Autodesk Inventor part; units mm, degrees
ref_plane "YZ Plane" through (0, 0, 0) normal (1, 0, 0) x (0, 1, 0)
ref_plane "XZ Plane" through (0, 0, 0) normal (0, 1, 0) x (-1, 0, 0)
ref_plane "XY Plane" through (0, 0, 0) normal (0, 0, 1) x (1, 0, 0)
sketch "Skizze1" plane through (0, 0, 0) normal (0, 1, 0) x (-1, 0, 0)
  line L0 (159.3398, 191.458) -> (9.3398, 191.458)
  line L1 (9.3398, 191.458) -> (9.3398, -108.542)
  line L2 (9.3398, -108.542) -> (159.3398, -108.542)
  line L3 (159.3398, -108.542) -> (159.3398, 191.458)
  point P0 (0, 0)
  dimension "d0" = 300
  dimension "d1" = 150
extrude "Extrusion1" add sketch "Skizze1" along normal blind 190
sketch "Skizze2" plane through (0, 190, 0) normal (0, 1, 0) x (1, 0, 0)
  line L0 (-9.3398, 108.542) -> (-159.3398, 108.542)
  line L1 (-159.3398, -191.458) -> (-9.3398, -191.458)
  line L2 (-9.3398, -191.458) -> (-9.3398, 108.542)
  line L3 (-9.3398, 108.542) -> (-159.3398, 108.542)
  line L4 (-159.3398, 108.542) -> (-159.3398, -191.458)
  line L5 (-9.3398, 108.542) -> (-89.3398, 108.542)
  line L6 (-89.3398, 108.542) -> (-89.3398, 48.542)
  line L7 (-69.3398, 28.542) -> (-9.3398, 28.542)
  line L8 (-9.3398, 28.542) -> (-9.3398, 108.542)
  line L9 (-9.3398, -191.458) -> (-9.3398, 108.542)
  line L10 (-9.3398, -191.458) -> (-89.3398, -191.458)
  line L11 (-89.3398, -191.458) -> (-89.3398, -131.458)
  line L12 (-69.3398, -111.458) -> (-9.3398, -111.458)
  line L13 (-9.3398, -111.458) -> (-9.3398, -191.458)
  arc A0 (-69.3398, -111.458) -> (-89.3398, -131.458) centre (-69.3398, -131.458) ccw
  arc A1 (-89.3398, 48.542) -> (-69.3398, 28.542) centre (-69.3398, 48.542) ccw
  point P0 (0, 0)
  point P1 (-89.3398, 28.542)
  point P2 (-89.3398, -111.458)
  dimension "d4" = 80
  dimension "d5" = 80
  dimension "d6" = 80
  dimension "d7" = 80
  dimension "d8" = 20
  dimension "d9" = 20
extrude "Extrusion2" cut sketch "Skizze2" against normal blind 20 contours L2 L7 A1 L6 L0 | L2 L1 L11 A0 L12
sketch "Skizze3" plane through (0, 170, 0) normal (0, 1, 0) x (1, 0, 0)
  line L0 (-9.3398, -111.458) -> (-9.3398, -191.458)
  line L1 (-69.3398, -111.458) -> (-9.3398, -111.458)
  arc A0 (-69.3398, -111.458) -> (-89.3398, -131.458) centre (-69.3398, -131.458) ccw
  line L2 (-89.3398, -191.458) -> (-89.3398, -131.458)
  line L3 (-9.3398, -191.458) -> (-89.3398, -191.458)
  line L4 (-9.3398, 108.542) -> (-9.3398, 28.542)
  line L5 (-89.3398, 108.542) -> (-9.3398, 108.542)
  line L6 (-89.3398, 48.542) -> (-89.3398, 108.542)
  arc A1 (-89.3398, 48.542) -> (-69.3398, 28.542) centre (-69.3398, 48.542) ccw
  line L7 (-9.3398, 28.542) -> (-69.3398, 28.542)
  circle A2 centre (-49.3398, -151.458) radius 7.5
  circle A3 centre (-49.3398, 68.542) radius 7.5
  point P0 (0, 0)
  dimension "d12" = 15
  dimension "d13" = 15
  dimension "d16" = 40
  dimension "d17" = 40
  dimension "d18" = 40
  dimension "d19" = 40
extrude "Extrusion3" add sketch "Skizze3" along normal blind 20 contours A2 | A3
properties part number "Baterie"
The model under review builds one solid part; all positions refer to its coordinate system, in mm. A direction names the side the tool comes from. Coordinates: 2 decimals unless noted, no trailing zeros. Write each loop counter-clockwise with the first axis right and the second up, starting at its lowest first coordinate (ties: lowest second). Pieces come first, ordered by that corner, then holes. Notation, with made-up numbers: (-17.5, 74) -> (26.5, 74) arc R14 ccw to (26.5, 92) -> close; hole circle Ø5 at (14.5, 30). An arc over 180 degrees is marked (long way). Answer in a Markdown table with one row per item.
1. Wall thickness on probe 1 along Y at (x, z) = (-34.5, -68.5); probe 2 along Z at (x, y) = (-35, 178): over which ranges is each line inside the solid? List them lowest first. Write a range as [from, to].
Answers below:
| item | result |
|---|---|
| probe 1 | y = [0, 170] |
| probe 2 | z = [-28.54, 111.46] |
2. We need section A-A, the plane x = -36. State the section outline as (y, z) points, and give its area (3 significant figures).
Answers below:
| item | result |
|---|---|
| outline | (0, -108.54) -> (170, -108.54) -> (170, -28.54) -> (190, -28.54) -> (190, 111.46) -> (170, 111.46) -> (170, 191.46) -> (0, 191.46) -> close |
| area | 53,800 mm^2 |
3. Draft analysis for pull direction Z (two halves, no side actions). For faces 6 (the cylindrical face through (-42.41, 179.86, 148.59)), 7 (the flat face through (-83, 94, -108.542)), 8 (the flat face through (-89.34, 180, -79)), state which applies: +Z half, -Z half, draft (parallel to the pull), parting line (faces both ways), or undercut.
Answers below:
| item | result |
|---|---|
| face 6 | undercut |
| face 7 | -Z half |
| face 8 | draft |
4. For faces 1 (the flat face through (-40, 180, 111.458)), 2 (the flat face through (-89.34, 180, 162)), 3 (the cylindrical face through (-83.64, 180.14, -34.56)), 4 (the cylindrical face through (-45.308, 179.86, -62.218)), 5 (the cylindrical face through (-83.326, 180.14, 117.161)), list the 3-axis set-ups (+Z, -Z, +X, -X, +Y, -Y) from which the entire face can be reached by the end or side of a thin tool; tool diameter is ignored.
Answers below:
| item | result |
|---|---|
| face 1 | +X, +Y |
| face 2 | +Z, +Y |
| face 3 | -Z, +X, +Y |
| face 4 | +Y |
| face 5 | +Z, +X, +Y |
5. Clearance check with flat-ended pins moving along their axes: pin 1 Ø8 at (x, z) = (-36, 122.5) entering from +Y; pin 2 Ø6 at (x, y) = (-43, 180) entering from +Z; pin 3 Ø10 at (x, y) = (-52, 178.5) entering from -Z. State where each tip first meets the part, or that it passes through.
Answers below:
| item | result |
|---|---|
| pin 1 | stops at y = 170 |
| pin 2 | stops at z = 158.17 |
| pin 3 | stops at z = -76.04 |
6. We need section B-B, the plane z = -41.5. State the section outline as (x, y) points, and give its area (3 significant figures).
Answers below:
| item | result |
|---|---|
| outline | (-159.34, 0) -> (-9.34, 0) -> (-9.34, 170) -> (-88.06, 170) -> (-88.06, 190) -> (-159.34, 190) -> close |
| area | 26,900 mm^2 |
